from build123d import *

# Parameters (mm, degrees)
EXTRUS_O1_DEPTH = 2.5
ESBO_O2_R       = 3
EXTRUS_O2_DEPTH = 20
ESBO_O3_R       = 5
EXTRUS_O3_DEPTH = 30
CHANFRO1_SIZE   = 0.5


with BuildPart() as part:
    # Esboço1 → Extrusão1 (new, symmetric)
    with BuildSketch(Plane.XY):
        Polygon((6.92820323, 0), (3.464101615, 6), (-3.464101615, 6), (-6.92820323, 0), (-3.464101615, -6), (3.464101615, -6), align=None)
    extrude(amount=EXTRUS_O1_DEPTH, both=True)

    # Esboço2 → Extrusão2 (add)
    with BuildSketch(Plane.XY.offset(2.5)):
        with Locations(Location((0, 0, 0), (0, 0, 180))):
            Circle(ESBO_O2_R)
    extrude(amount=EXTRUS_O2_DEPTH)

    # Esboço3 → Extrusão3 (add)
    with BuildSketch(Plane(origin=(0, 0, -2.5), x_dir=(-1, 0, 0), z_dir=(0, 0, -1))):
        Circle(ESBO_O3_R)
    extrude(amount=EXTRUS_O3_DEPTH)

    # Chanfro1
    chanfro1_edges = [part.edges().sort_by_distance(p)[0] for p in [
        (3, 0, 22.5),
        (5, 0, -32.5),
    ]]
    chamfer(chanfro1_edges, length=CHANFRO1_SIZE)


solid = part.part
For this review, take the finished solid that the model builds, in its own axes (mm). A direction names the side the tool comes from. Coordinates: 2 decimals unless noted, no trailing zeros. Order: outer loops, then holes, each group sorted by start corner. A loop starts at its lowest first (then second) coordinate and runs counter-clockwise, first axis right, second up. Notation, with made-up numbers: (42, 3.5) - (99, 3.5) arc R18 ccw to (99, 13.5) - close; hole circle Ø4 at (51.25, -18). An arc over 180 degrees is marked (long way). Answer as CSV lines item,"result". Start each with the question number.
1) Machinability: for faces 1 (the flat face through (1, 3, 2.5)), 2 (the flat face through (0, 0, -32.5)), 3 (the cylindrical face through (1.08, -4.88, -17.04)), which of the approach directions +Z, -Z, +X, -X, +Y, -Y give a long, thin tool a straight path to every point of the face, cutting with its end or side? Answer none if there is none.
2) To check wall thickness, follow line 1 along Z through (x, y) = (0.5, -3.75); line 2 along Z through (x, y) = (-3.25, 4.75); line 3 along X through (y, z) = (-4, -14.5). State the ranges of each line that lie inside material, in increasing order. Write a range as [from, to].
3) Add section C-C (z = 15). State the section outline as (x, y) points, then the cut area to 3 significant figures.
4) Add section A-A (x = 0). State the section outline as (y, z) points, then the cut area to 4 significant figures.
5) Insertion check: P1, Ø2, axis at y = 4, z = -13.5, coming from the -X side; P2, Ø6, axis at x = -5, z = -9.5, coming from the -Y side; P3, Ø5, axis at x = 4.5, z = -15.5, coming from the +Y side. Each pin has a flat end and moves straight along its axis. Give the tip position at first contact, or say it passes through.
6) Add section B-B (z = -3). State the section outline as (x, y) points.
Result:
1,face 1,"+Z"
1,face 2,"-Z, +X, -X, +Y, -Y"
1,face 3,"-Z"
2,line 1,"[-32.5, 2.5]"
2,line 2,"[-2.5, 2.5]"
2,line 3,"[-3, 3]"
3,outline,"circle Ø6 at (0, 0)"
3,area,"28.3 mm^2"
4,outline,"(-6, -2.5) - (-5, -2.5) - (-5, -32) - (-4.5, -32.5) - (4.5, -32.5) - (5, -32) - (5, -2.5) - (6, -2.5) - (6, 2.5) - (3, 2.5) - (3, 22) - (2.5, 22.5) - (-2.5, 22.5) - (-3, 22) - (-3, 2.5) - (-6, 2.5) - close"
4,area,"479.5 mm^2"
5,P1,"x = -4"
5,P2,"y = -4.58"
5,P3,"y = 4.58"
6,outline,"circle Ø10 at (0, 0)"
